from build123d import *

# Parameters (mm, degrees)
F0_W     = 38.1
F0_H     = 88.9
F1_DEPTH = 971.64906
F3_DEPTH = 25.4
F5_DEPTH = 25.4


with BuildPart() as f1:
    # F0 (on Front) → F1 (new body)
    with BuildSketch(Plane.XZ):
        Rectangle(F0_W, F0_H)
    extrude(amount=F1_DEPTH)

    # F2 (on Right) → F3 (cut, symmetric)
    with BuildSketch(Plane.YZ):
        Polygon((-972.82, -44.45), (-948.944, 44.45), (-972.82, 44.45), align=None)
    extrude(amount=F3_DEPTH, both=True, mode=Mode.SUBTRACT)

    # F4 (on Right) → F5 (cut, symmetric)
    with BuildSketch(Plane.YZ):
        Polygon((-23.876, -44.45), (0, -44.45), (0, 44.45), (-39.37, 44.45), (-2.688901, 34.621329), align=None)
    extrude(amount=F5_DEPTH, both=True, mode=Mode.SUBTRACT)


solid = f1.part
Model file for the job. Use its own axes, mm. Round coordinates to 2 decimals unless told otherwise and drop trailing zeros. Order: outer loops, then holes, each group sorted by start corner. A loop starts at its lowest first (then second) coordinate and runs counter-clockwise, first axis right, second up. Notation, with made-up numbers: M -13,-6 L 10,-6 A17 ccw 10,20 Z; hole C -4.75,73.25 d4. An arc over 180 degrees is marked long. Write each question's results on one line, items separated by ' | '. Start each with the question number.
(1) Saw through at B-B, the plane z = -11. Give the cut face in (x, y), then the cut area to 3 significant figures.
(2) Drop flat-ended pins along their axis: pin 1 (1.5 mm diameter, centred on x = 5.5, z = 35.5, fed in from -Y); pin 2 (12 mm diameter, centred on x = 8, z = 23, fed in from +Y); pin 3 (5 mm diameter, centred on x = -15, z = -19, fed in from -Y). Give the stop position or say it passes through.
(3) Probe probe 1 along Y at (x, z) = (0.5, 6); probe 2 along Y at (x, z) = (3, 28.5). List the from-to ranges inside material, lowest first. Write a range as from..to.
(4) Saw through at A-A, the plane x = 11.5. Give the cut face in (y, z), then the cut area to 3 significant figures.
Established:
1) outline: M -19.05,-963.84 L 19.05,-963.84 L 19.05,-14.91 L -19.05,-14.91 Z | area: 36,200 mm^2
2) pin 1: stops at y = -951.55 | pin 2: stops at y = -4.2 | pin 3: stops at y = -966.66
3) probe 1: y = -959.27..-10.36 | probe 2: y = -953.23..-4.33
4) outline: M -971.65,-44.45 L -23.88,-44.45 L -2.69,34.62 L -39.37,44.45 L -948.94,44.45 L -971.65,-40.09 Z | area: 84,200 mm^2
